Build history of the part. All positions in model axes, mm. Face numbers are marked on the shaded views. A direction names the side the tool comes from. Round coordinates to 2 decimals unless told otherwise and drop trailing zeros. Order: outer loops, then holes, each group sorted by start corner. A loop starts at its lowest first (then second) coordinate and runs counter-clockwise, first axis right, second up. Notation, with made-up numbers: (4.25, 84.5) -> (10.25, 84.5) arc R33 cw to (10.25, 112.5) -> close; hole circle Ø7 at (80.25, 37.25). An arc over 180 degrees is marked (long way). Answer as CSV lines item,"result". Start each with the question number.
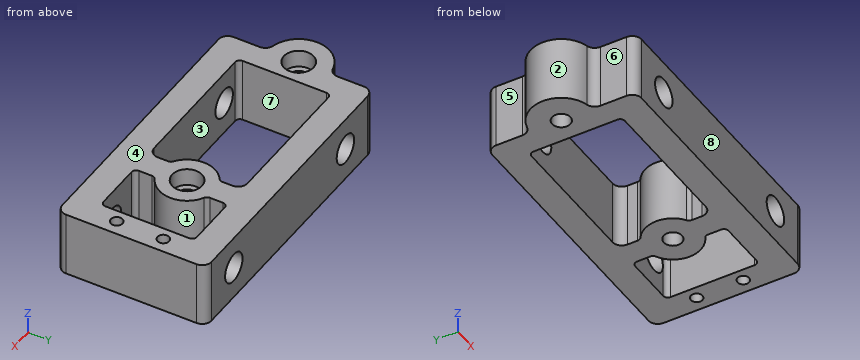
```python
from build123d import *

# Parameters (mm, degrees)
SKETCH1_W           = 93.6625
SKETCH1_H           = 40.64
SKETCH1_R           = 2.4892
SKETCH1_R_2         = 1.5875
BOSS_EXTRUDE1_DEPTH = 17.78
SKETCH6_R           = 3.96875
CUT_EXTRUDE4_DEPTH  = 41.64
CUT_EXTRUDE3_DEPTH  = 17.78
FILLET1_R           = 2.54
SKETCH3_R           = 4.064
CUT_EXTRUDE5_DEPTH  = 4.7752
SKETCH7_W           = 9.113549332
SKETCH7_H           = 21.245092044
CUT_EXTRUDE6_DEPTH  = 18.78
SKETCH8_W           = 17.78
SKETCH8_H           = 25.4
CUT_EXTRUDE7_DEPTH  = 17.78
FILLET2_R           = 1.27


with BuildPart() as part:
    # Sketch1 → Boss-Extrude1 (new body)
    with BuildSketch(Plane.XY):
        with Locations((-46.83125, 0)):
            Rectangle(SKETCH1_W, SKETCH1_H)
        with Locations((-84.93125, 0)):
            Circle(SKETCH1_R, mode=Mode.SUBTRACT)
        with Locations((-34.13125, 0)):
            Circle(SKETCH1_R, mode=Mode.SUBTRACT)
        with Locations((-12.7, 6.35)):
            Circle(SKETCH1_R_2, mode=Mode.SUBTRACT)
        with Locations((-12.7, -6.35)):
            Circle(SKETCH1_R_2, mode=Mode.SUBTRACT)
    extrude(amount=-BOSS_EXTRUDE1_DEPTH)

    # Sketch6 → Cut-Extrude4 (cut, through all)
    with BuildSketch(Plane(origin=(0, 20.32, 0), x_dir=(1, 0, 0), z_dir=(0, 1, 0))):
        with Locations((-72.23125, 8.89)):
            Circle(SKETCH6_R)
        with Locations((-21.43125, 8.89)):
            Circle(SKETCH6_R)
    extrude(amount=-CUT_EXTRUDE4_DEPTH, mode=Mode.SUBTRACT)

    # Sketch5 → Cut-Extrude3 (cut)
    with BuildSketch(Plane.XY):
        with BuildLine():
            Line((-93.6625, -20.32), (-93.6625, 20.32))
            Line((-93.6625, 20.32), (-84.93125, 20.32))
            Line((-84.93125, 20.32), (-84.93125, 10.622546022))
            ThreePointArc((-84.93125, 10.622546022), (-85.477262526, 9.049137635), (-86.880552326, 8.152186482))
            ThreePointArc((-86.880552326, 8.152186482), (-93.31325, 0), (-86.880552326, -8.152186482))
            ThreePointArc((-86.880552326, -8.152186482), (-85.477262526, -9.049137635), (-84.93125, -10.622546022))
            Line((-84.93125, -10.622546022), (-84.93125, -20.32))
            Line((-84.93125, -20.32), (-93.6625, -20.32))
        make_face()
        with BuildLine():
            Line((0, -20.32), (0, 20.32))
            Line((0, 20.32), (-8.73125, 20.32))
            Line((-8.73125, 20.32), (-8.73125, 10.622546022))
            ThreePointArc((-8.73125, 10.622546022), (-8.185237474, 9.049137635), (-6.781947674, 8.152186482))
            ThreePointArc((-6.781947674, 8.152186482), (-0.34925, 0), (-6.781947674, -8.152186482))
            ThreePointArc((-6.781947674, -8.152186482), (-8.185237474, -9.049137635), (-8.73125, -10.622546022))
            Line((-8.73125, -10.622546022), (-8.73125, -20.32))
            Line((-8.73125, -20.32), (0, -20.32))
        make_face()
    extrude(amount=-CUT_EXTRUDE3_DEPTH, mode=Mode.SUBTRACT)

    # Fillet1
    fillet1_edges = [part.edges().sort_by_distance(p)[0] for p in [
        (-84.93125, 20.32, -8.89),
        (-84.93125, -20.32, -8.89),
        (-8.73125, 20.32, -8.89),
        (-8.73125, -20.32, -8.89),
    ]]
    fillet(fillet1_edges, radius=FILLET1_R)

    # Sketch3 → Cut-Extrude5 (cut)
    with BuildSketch(Plane.XY):
        with Locations((-84.93125, 0)):
            Circle(SKETCH3_R)
        with Locations((-34.13125, 0)):
            Circle(SKETCH3_R)
    extrude(amount=-CUT_EXTRUDE5_DEPTH, mode=Mode.SUBTRACT)

    # Sketch7 → Cut-Extrude6 (cut, through all)
    with BuildSketch(Plane.XY):
        with BuildLine():
            Line((-37.842518981, 10.16), (-37.842518981, 6.655139559))
            ThreePointArc((-37.842518981, 6.655139559), (-41.75125, 0), (-37.842518981, -6.655139559))
            Line((-37.842518981, -6.655139559), (-37.842518981, -10.16))
            ThreePointArc((-37.842518981, -10.16), (-38.586467757, -11.956051224), (-40.382518981, -12.7))
            Line((-40.382518981, -12.7), (-60.702518981, -12.7))
            ThreePointArc((-60.702518981, -12.7), (-62.498570205, -11.956051224), (-63.242518981, -10.16))
            Line((-63.242518981, -10.16), (-63.242518981, 10.16))
            ThreePointArc((-63.242518981, 10.16), (-62.498570205, 11.956051224), (-60.702518981, 12.7))
            Line((-60.702518981, 12.7), (-40.382518981, 12.7))
            ThreePointArc((-40.382518981, 12.7), (-38.586467757, 11.956051224), (-37.842518981, 10.16))
        make_face()
        with Locations((-4.174475334, 0)):
            Rectangle(SKETCH7_W, SKETCH7_H)
    extrude(amount=-CUT_EXTRUDE6_DEPTH, mode=Mode.SUBTRACT)

    # Sketch8 → Cut-Extrude7 (cut)
    with BuildSketch(Plane.XY):
        with Locations((-69.592518981, 0)):
            Rectangle(SKETCH8_W, SKETCH8_H)
        with BuildLine():
            Line((-31.316413003, 12.7), (-16.076413003, 12.7))
            Line((-16.076413003, 12.7), (-16.076413003, -12.7))
            Line((-16.076413003, -12.7), (-31.316413003, -12.7))
            Line((-31.316413003, -12.7), (-31.316413003, -7.046567735))
            ThreePointArc((-31.316413003, -7.046567735), (-26.543271075, 0), (-31.316413003, 7.046567735))
            Line((-31.316413003, 7.046567735), (-31.316413003, 12.7))
        make_face()
    extrude(amount=-CUT_EXTRUDE7_DEPTH, mode=Mode.SUBTRACT)

    # Fillet2
    fillet2_edges = [part.edges().sort_by_distance(p)[0] for p in [
        (-37.842518981, 6.655139559, -8.89),
        (-37.842518981, -6.655139559, -8.89),
        (-78.482518981, 12.7, -8.89),
        (-78.482518981, -12.7, -8.89),
        (-16.076413003, -12.7, -8.89),
        (-31.316413003, 12.7, -8.89),
        (-31.316413003, -12.7, -8.89),
        (-16.076413003, 12.7, -8.89),
        (-31.316413003, 7.046567735, -8.89),
        (-31.316413003, -7.046567735, -8.89),
    ]]
    fillet(fillet2_edges, radius=FILLET2_R)


solid = part.part
```
Q1. Probe L1, parallel to X at y = 15, z = -8.89; L2, parallel to Y at x = -12.7, z = -6.5; L3, parallel to X at y = -12.5, z = -6.5. List the from-to ranges inside material, lowest first.
Q2. Flat gauge pins, fed straight in: pin 1 Ø1.5 at (y, z) = (-5.5, -6.5) entering from -X; pin 2 Ø6 at (y, z) = (-9, -10.5) entering from -X; pin 3 Ø5 at (x, y) = (-79.5, 8) entering from +Z; pin 4 Ø6.5 at (x, y) = (-84.93, 0) entering from +Z. Where does each tip first touch, or does it go through?
Q3. Two-plate mould, pull along X, no slides. Class the marked faces 1, 2, 3 and 4: +X half, -X half, draft (parallel to the pull), parting line (faces both ways), or undercut.
Q4. Slice it at A-A, the plane x = -12.7. Write the cut outline in (y, z).
Q5. Which spindle directions (+Z, -Z, +X, -X, +Y, -Y) get a long thin tool onto all of the face, cutting with end or side? Do the marked faces 5, 6, 7 and 8. Say none if no direction does.
Q6. Slice it at C-C, the plane y = 14. Write the cut outline in (x, z), plus the area to 3 significant figures.
Q7. Slice it at D-D, the plane z = -8.89. Count the separate pieces of the cut face and the enclosed holes in it, plus the area to 3 significant figures.
Q8. Slice it at B-B, the plane x = -61.5. Write the cut outline in (y, z), plus the area to 3 significant figures.
Solutions:
1,L1,"x = -84.93 to -76.2, -68.26 to -25.4, -17.46 to -8.73"
1,L2,"y = -20.32 to -7.94, -4.76 to 4.76, 7.94 to 20.32"
1,L3,"x = -84.93 to -77.9, -39.39 to -30.73, -16.66 to -8.73"
2,pin 1,"stops at x = -91.84"
2,pin 2,"stops at x = -90.78"
2,pin 3,"stops at z = 0"
2,pin 4,"stops at z = -4.78"
3,face 1,"undercut"
3,face 2,"-X half"
3,face 3,"undercut"
3,face 4,"draft"
4,outline,"(-20.32, -17.78) -> (-7.94, -17.78) -> (-7.94, 0) -> (-20.32, 0) -> close; (-4.76, -17.78) -> (4.76, -17.78) -> (4.76, 0) -> (-4.76, 0) -> close; (7.94, -17.78) -> (20.32, -17.78) -> (20.32, 0) -> (7.94, 0) -> close"
5,face 5,"+Z, -Z, -X, +Y"
5,face 6,"+Z, -Z, -X, -Y"
5,face 7,"+Z, -Z"
5,face 8,"+Z, -Z, +X, -X, -Y"
6,outline,"(-84.93, -17.78) -> (-8.73, -17.78) -> (-8.73, 0) -> (-84.93, 0) -> close; hole circle Ø7.94 at (-72.23, -8.89); hole circle Ø7.94 at (-21.43, -8.89)"
6,area,"1,260 mm2"
7,separate pieces,"3"
7,enclosed holes,"4"
7,area,"1,580 mm2"
8,outline,"(-20.32, -17.78) -> (-12.7, -17.78) -> (-12.7, 0) -> (-20.32, 0) -> close; (12.7, -17.78) -> (20.32, -17.78) -> (20.32, 0) -> (12.7, 0) -> close"
8,area,"271 mm2"
